Geometry: final body of the model. Coordinates: model frame, mm. A direction names the side the tool comes from. Give positions to 0.01 mm unless a question says otherwise; leave off trailing zeros. Order: outer loops, then holes, each group sorted by start corner. A loop starts at its lowest first (then second) coordinate and runs counter-clockwise, first axis right, second up. Notation, with made-up numbers: (-12, -24.5) - (37, -24.5) arc R10 ccw to (37, -15.5) - close; hole circle Ø11 at (69, -39). An arc over 180 degrees is marked (long way). One line per question, with ' | ' between items. Start each with the question number.
from build123d import *

# Parameters (mm, degrees)
SKETCH_1_W                = 60
SKETCH_1_H                = 4
EXTRUDE_1_DEPTH           = 64
SKETCH_2_W                = 4
SKETCH_2_H                = 64
EXTRUDE_2_DEPTH           = 50
FILLET_1_R                = 10
CUT_EXTRUDE_1_REACH       = 92.324
SKETCH_4_W                = 11
SKETCH_4_H                = 52
EXTRUDE_3_DEPTH           = 4
EXTRUDE_4_DEPTH           = 5
EXTRUDE_4_DRAFT           = 4
EXTRUDE_4_PROFILE_2_DEPTH = 5
EXTRUDE_4_PROFILE_2_DRAFT = 4
FILLET_2_R                = 4
EXTRUDE_5_DEPTH           = 5.2
EXTRUDE_6_DEPTH           = 5
FILLET_3_R                = 1
SKETCH_8_W                = 4
SKETCH_8_H                = 22
EXTRUDE_7_DEPTH           = 12
FILLET_4_R                = 5
CUT_EXTRUDE_2_REACH       = 96.252


with BuildPart() as part:
    # Sketch 1 → Extrude 1 (new body)
    with BuildSketch(Plane(origin=(0, 0, 0), x_dir=(1, 0, 0), z_dir=(0, 1, 0))):
        with Locations((-88.556547212, 28.436915988)):
            Rectangle(SKETCH_1_W, SKETCH_1_H)
    extrude(amount=EXTRUDE_1_DEPTH)

    # Sketch 2 → Extrude 2 (add)
    with BuildSketch(Plane.XY.offset(-26.436915988)):
        with Locations((-116.556547212, 32)):
            Rectangle(SKETCH_2_W, SKETCH_2_H)
    extrude(amount=EXTRUDE_2_DEPTH)

    # Fillet 1
    fillet_1_edges = [part.edges().sort_by_distance(p)[0] for p in [
        (-58.556547212, 64, -28.436915988),
        (-116.556547212, 0, 23.563084012),
        (-116.556547212, 64, 23.563084012),
        (-58.556547212, 0, -28.436915988),
    ]]
    fillet(fillet_1_edges, radius=FILLET_1_R)

    # Sketch 3 → Cut-Extrude 1 (cut, up to next)
    with BuildSketch(Plane(origin=(-114.556547212, 0, 0), x_dir=(0, 0, -1), z_dir=(1, 0, 0)), mode=Mode.PRIVATE) as cut_extrude_1_sk1:
        with BuildLine():
            Line((-17.563084012, 54), (-17.563084012, 10))
            ThreePointArc((-17.563084012, 10), (-16.391511137, 7.171572875), (-13.563084012, 6))
            Line((-13.563084012, 6), (20.436915988, 6))
            Line((20.436915988, 6), (20.436915988, 58))
            Line((20.436915988, 58), (-13.563084012, 58))
            ThreePointArc((-13.563084012, 58), (-16.391511137, 56.828427125), (-17.563084012, 54))
        make_face()
    cut_extrude_1_tool1 = extrude(cut_extrude_1_sk1.sketch, amount=-CUT_EXTRUDE_1_REACH, mode=Mode.PRIVATE) & part.part
    add(cut_extrude_1_tool1.solids().sort_by_distance((-114.556547, 32, -1.500062))[0], mode=Mode.SUBTRACT)


with BuildPart() as body_2:
    # Sketch 4 → Extrude 3 (new body)
    with BuildSketch(Plane.ZY.offset(118.556547212)):
        with Locations((-14.936915988, 32)):
            Rectangle(SKETCH_4_W, SKETCH_4_H)
    extrude(amount=-EXTRUDE_3_DEPTH)


with BuildPart() as extrude_4_tool:
    # Sketch 5 → Extrude 4 (with draft: the straight prism first)
    with BuildSketch(Plane(origin=(-114.556547212, 0, 0), x_dir=(0, 0, -1), z_dir=(1, 0, 0))):
        with BuildLine():
            ThreePointArc((12.936915988, 53.2), (11.736915988, 52), (12.936915988, 50.8))
            Line((12.936915988, 50.8), (16.936915988, 50.8))
            ThreePointArc((16.936915988, 50.8), (18.136915988, 52), (16.936915988, 53.2))
            Line((16.936915988, 53.2), (12.936915988, 53.2))
        make_face()
    extrude(amount=EXTRUDE_4_DEPTH)
    # Extrude 4: the draft: its side faces are tilted about the plane it starts from
    extrude_4_sides = [extrude_4_tool.faces().sort_by_distance(p)[0] for p in [
        (-112.056547212, 52, -18.136915988),
        (-112.056547212, 53.2, -14.936915988),
        (-112.056547212, 52, -11.736915988),
        (-112.056547212, 50.8, -14.936915988),
    ]]
    draft(extrude_4_sides, Plane(origin=(-114.556547212, 0, 0), x_dir=(0, 0, -1), z_dir=(1, 0, 0)), EXTRUDE_4_DRAFT)


with BuildPart() as part_1:
    add(part.part)

    # Extrude 4: add extrude_4_tool
    add(extrude_4_tool.part)

    add(body_2.part)  # Extrude 4 merges body 2


with BuildPart() as extrude_4_profile_2_tool:
    # Sketch 5 → Extrude 4 profile 2 (with draft: the straight prism first)
    with BuildSketch(Plane(origin=(-114.556547212, 0, 0), x_dir=(0, 0, -1), z_dir=(1, 0, 0))):
        with BuildLine():
            ThreePointArc((12.936915988, 13.2), (11.736915988, 12), (12.936915988, 10.8))
            Line((12.936915988, 10.8), (16.936915988, 10.8))
            ThreePointArc((16.936915988, 10.8), (18.136915988, 12), (16.936915988, 13.2))
            Line((16.936915988, 13.2), (12.936915988, 13.2))
        make_face()
    extrude(amount=EXTRUDE_4_PROFILE_2_DEPTH)
    # Extrude 4 profile 2: the draft: its side faces are tilted about the plane it starts from
    extrude_4_profile_2_sides = [extrude_4_profile_2_tool.faces().sort_by_distance(p)[0] for p in [
        (-112.056547212, 12, -11.736915988),
        (-112.056547212, 10.8, -14.936915988),
        (-112.056547212, 12, -18.136915988),
        (-112.056547212, 13.2, -14.936915988),
    ]]
    draft(extrude_4_profile_2_sides, Plane(origin=(-114.556547212, 0, 0), x_dir=(0, 0, -1), z_dir=(1, 0, 0)), EXTRUDE_4_PROFILE_2_DRAFT)


with BuildPart() as part_2:
    add(part_1.part)

    # Extrude 4 profile 2: add extrude_4_profile_2_tool
    add(extrude_4_profile_2_tool.part)

    # Fillet 2
    fillet_2_edges = [part_2.edges().sort_by_distance(p)[0] for p in [
        (-116.556547212, 58, -9.436915988),
        (-116.556547212, 6, -9.436915988),
    ]]
    fillet(fillet_2_edges, radius=FILLET_2_R)

    # Sketch 6 → Extrude 5 (add)
    with BuildSketch(Plane(origin=(0, 0, -30.436915988), x_dir=(-1, 0, 0), z_dir=(0, 0, -1))):
        with BuildLine():
            Line((60.956547212, 54.4), (63.456547212, 54.4))
            ThreePointArc((63.456547212, 54.4), (65.856547212, 52), (63.456547212, 49.6))
            Line((63.456547212, 49.6), (60.956547212, 49.6))
            ThreePointArc((60.956547212, 49.6), (58.556547212, 52), (60.956547212, 54.4))
        make_face()
        with BuildLine():
            Line((100.956547212, 54.4), (103.456547212, 54.4))
            ThreePointArc((103.456547212, 54.4), (105.856547212, 52), (103.456547212, 49.6))
            Line((103.456547212, 49.6), (100.956547212, 49.6))
            ThreePointArc((100.956547212, 49.6), (98.556547212, 52), (100.956547212, 54.4))
        make_face()
        with BuildLine():
            Line((100.956547212, 14.4), (103.456547212, 14.4))
            ThreePointArc((103.456547212, 14.4), (105.856547212, 12), (103.456547212, 9.6))
            Line((103.456547212, 9.6), (100.956547212, 9.6))
            ThreePointArc((100.956547212, 9.6), (98.556547212, 12), (100.956547212, 14.4))
        make_face()
        with BuildLine():
            Line((60.956547212, 14.4), (63.456547212, 14.4))
            ThreePointArc((63.456547212, 14.4), (65.856547212, 12), (63.456547212, 9.6))
            Line((63.456547212, 9.6), (60.956547212, 9.6))
            ThreePointArc((60.956547212, 9.6), (58.556547212, 12), (60.956547212, 14.4))
        make_face()
    extrude(amount=EXTRUDE_5_DEPTH)

    # Sketch 7 → Extrude 6 (add)
    with BuildSketch(Plane(origin=(0, 0, -35.636915988), x_dir=(-1, 0, 0), z_dir=(0, 0, -1))):
        with BuildLine():
            Line((60.956547212, 54.4), (69.756547212, 54.4))
            ThreePointArc((69.756547212, 54.4), (72.156547212, 52), (69.756547212, 49.6))
            Line((69.756547212, 49.6), (60.956547212, 49.6))
            ThreePointArc((60.956547212, 49.6), (58.556547212, 52), (60.956547212, 54.4))
        make_face()
        with BuildLine():
            Line((100.956547212, 54.4), (109.756547212, 54.4))
            ThreePointArc((109.756547212, 54.4), (112.156547212, 52), (109.756547212, 49.6))
            Line((109.756547212, 49.6), (100.956547212, 49.6))
            ThreePointArc((100.956547212, 49.6), (98.556547212, 52), (100.956547212, 54.4))
        make_face()
        with BuildLine():
            Line((100.956547212, 14.4), (109.756547212, 14.4))
            ThreePointArc((109.756547212, 14.4), (112.156547212, 12), (109.756547212, 9.6))
            Line((109.756547212, 9.6), (100.956547212, 9.6))
            ThreePointArc((100.956547212, 9.6), (98.556547212, 12), (100.956547212, 14.4))
        make_face()
        with BuildLine():
            Line((60.956547212, 14.4), (69.756547212, 14.4))
            ThreePointArc((69.756547212, 14.4), (72.156547212, 12), (69.756547212, 9.6))
            Line((69.756547212, 9.6), (60.956547212, 9.6))
            ThreePointArc((60.956547212, 9.6), (58.556547212, 12), (60.956547212, 14.4))
        make_face()
    extrude(amount=EXTRUDE_6_DEPTH)

    # Fillet 3
    fillet_3_edges = [part_2.edges().sort_by_distance(p)[0] for p in [
        (-66.606547212, 49.6, -35.636915988),
        (-72.156547212, 52, -35.636915988),
        (-66.606547212, 54.4, -35.636915988),
        (-106.606547212, 49.6, -35.636915988),
        (-112.156547212, 52, -35.636915988),
        (-106.606547212, 54.4, -35.636915988),
        (-106.606547212, 9.6, -35.636915988),
        (-112.156547212, 12, -35.636915988),
        (-106.606547212, 14.4, -35.636915988),
        (-66.606547212, 9.6, -35.636915988),
        (-72.156547212, 12, -35.636915988),
        (-66.606547212, 14.4, -35.636915988),
    ]]
    fillet(fillet_3_edges, radius=FILLET_3_R)

    # Sketch 8 → Extrude 7 (add)
    with BuildSketch(Plane.XZ):
        with Locations((-116.556547212, -19.436915988)):
            Rectangle(SKETCH_8_W, SKETCH_8_H)
    extrude(amount=EXTRUDE_7_DEPTH)

    # Fillet 4
    fillet_4_edges = [part_2.edges().sort_by_distance(p)[0] for p in [
        (-116.556547212, 0, -8.436915988),
        (-116.556547212, -12, -8.436915988),
    ]]
    fillet(fillet_4_edges, radius=FILLET_4_R)

    # Sketch 9 → Cut-Extrude 2 (cut, up to next)
    with BuildSketch(Plane(origin=(-114.556547212, 0, 0), x_dir=(0, 0, -1), z_dir=(1, 0, 0)), mode=Mode.PRIVATE) as cut_extrude_2_sk1:
        with BuildLine():
            Line((14.436915988, -2), (24.436915988, -2))
            ThreePointArc((24.436915988, -2), (28.436915988, -6), (24.436915988, -10))
            Line((24.436915988, -10), (14.436915988, -10))
            ThreePointArc((14.436915988, -10), (10.436915988, -6), (14.436915988, -2))
        make_face()
    cut_extrude_2_tool1 = extrude(cut_extrude_2_sk1.sketch, amount=-CUT_EXTRUDE_2_REACH, mode=Mode.PRIVATE) & part_2.part
    add(cut_extrude_2_tool1.solids().sort_by_distance((-114.556547, -6, -19.436916))[0], mode=Mode.SUBTRACT)


solid = part_2.part
(1) Cut plane D-D, the plane x = -90. Return the cut outline in (y, z), plus the area to 3 significant figures.
(2) Pull-direction query (Z, two-part tool) for faces 1 (the flat face through (-92, 0, -28)), 2 (the cylindrical face through (-116.529, 2.852, 20.556)), 3 (the conical face through (-112.092, 51.977, -17.964)); classes: +Z half, -Z half, draft (parallel to the pull), parting line (faces both ways), or undercut.
(3) Contact query for flat-ended pins moving along their axis: P1, Ø0.9, axis at y = 11.5, z = -15.5, coming from the +X side; P2, Ø5, axis at y = -2, z = -23.5, coming from the +X side; P3, Ø1.4, axis at x = -107, y = 12.5, coming from the +Z side. Output: stop coordinate, or through.
(4) Access query for faces 4 (the flat face through (-117, 32, 17.563)), 5 (the cylindrical face through (-65.856, 52.053, -33.494)), 6 (the flat face through (-112.092, 50.972, -14.909)), 7 (the flat face through (-64, 49.6, -38)). Directions: +Z, -Z, +X, -X, +Y, -Y. A direction counts if a zero-diameter tool reaches every point of the face in a straight line with its end or side. Return the directions, or none.
(5) Cut plane A-A, the plane y = 20. Return the cut outline in (x, z), plus the area to 3 significant figures.
(6) Cut plane C-C, the plane y = -6. Return the cut outline in (x, z), plus the area to 3 significant figures.
(7) Material intervals for line 1 along Z through (x, y) = (-91.5, 11); line 2 along X through (y, z) = (22, 18); line 3 along Z through (x, y) = (-66.5, 10), sorted ascending. Write a range as from..to.
(8) Cut plane B-B, the plane z = 6.5. Return the cut outline in (x, y).
Results are:
1) outline: (0, -30.44) - (64, -30.44) - (64, -26.44) - (0, -26.44) - close | area: 256 mm2
2) face 1: draft | face 2: +Z half | face 3: undercut
3) P1: x = -109.56 | P2: x = -114.56 | P3: z = -26.44
4) face 4: +X, -X | face 5: none | face 6: +Z, +X | face 7: -Z, +X, -X
5) outline: (-118.56, -30.44) - (-58.56, -30.44) - (-58.56, -26.44) - (-114.56, -26.44) - (-114.56, -9.44) - (-118.56, -9.44) - close; (-118.56, 17.56) - (-114.56, 17.56) - (-114.56, 23.56) - (-118.56, 23.56) - close | area: 332 mm2
6) outline: (-118.56, -30.44) - (-114.56, -30.44) - (-114.56, -28.44) - (-118.56, -28.44) - close; (-118.56, -10.44) - (-114.56, -10.44) - (-114.56, -8.44) - (-118.56, -8.44) - close | area: 16.0 mm2
7) line 1: -30.44..-26.44 | line 2: -118.56..-114.56 | line 3: -40.64..-35.84, -30.44..-26.44
8) outline: (-118.56, 0) - (-114.56, 0) - (-114.56, 6) - (-118.56, 6) - close; (-118.56, 58) - (-114.56, 58) - (-114.56, 64) - (-118.56, 64) - close
